Read the model definition and answer for the solid it produces. Units are mm, in the model's axes. A direction names the side the tool comes from. Give positions to 0.01 mm unless a question says otherwise; leave off trailing zeros. Loops run counter-clockwise (first coordinate to the right, second up) from the corner with the lowest first, then second, coordinate; pieces in that order, holes last. Notation, with made-up numbers: (9.25, -7) - (59.25, -7) arc R24 ccw to (59.25, 18) - close; hole circle Ø3 at (39.5, 45). An arc over 180 degrees is marked (long way). Write item = value, one per line. Start each with the question number.
from build123d import *
from build123d.topology import SkipClean

# Parameters (mm, degrees)
BOSS_EXTRUDE1_DEPTH             = 2
BOSS_EXTRUDE2_START             = -13.63
BOSS_EXTRUDE2_DEPTH             = 13.63
BOSS_EXTRUDE3_DEPTH             = 2
SKETCH5_W                       = 22.5
SKETCH5_H                       = 6.1
CUT_EXTRUDE1_DEPTH              = 28.613527482
BOSS_EXTRUDE4_REACH             = 29.614
SKETCH6_W                       = 22.5
SKETCH6_H                       = 3
BOSS_EXTRUDE4_DIRECTION_2_REACH = 29.614
FILLET1_R                       = 2


with BuildPart() as part:
    # Sketch1 → Boss-Extrude1 (new body)
    with BuildSketch(Plane(origin=(0, 0, 0), x_dir=(1, 0, 0), z_dir=(0, 1, 0))):
        with BuildLine():
            Line((2, 0), (20.5, 0))
            ThreePointArc((20.5, 0), (21.914213562, 0.585786438), (22.5, 2))
            Line((22.5, 2), (22.5, 5))
            ThreePointArc((22.5, 5), (21.914213562, 6.414213562), (20.5, 7))
            Line((20.5, 7), (2, 7))
            ThreePointArc((2, 7), (0.585786438, 6.414213562), (0, 5))
            Line((0, 5), (0, 2))
            ThreePointArc((0, 2), (0.585786438, 0.585786438), (2, 0))
        make_face()
    extrude(amount=BOSS_EXTRUDE1_DEPTH)

    # Sketch2 → Boss-Extrude2 (add)
    with SkipClean():  # the faces are left unmerged after this step: merging them gives an invalid solid
        with BuildSketch(Plane(origin=(0, 2, 0), x_dir=(1, 0, 0), z_dir=(0, 1, 0)).offset(BOSS_EXTRUDE2_START)):
            with BuildLine():
                Line((22.5, 5), (22.5, 2))
                ThreePointArc((22.5, 2), (22.202938637, 0.951191152), (21.4, 0.21394289))
                Line((21.4, 0.21394289), (21.4, 3.1))
                ThreePointArc((21.4, 3.1), (20.521320344, 5.221320344), (18.4, 6.1))
                Line((18.4, 6.1), (4.1, 6.1))
                ThreePointArc((4.1, 6.1), (1.978679656, 5.221320344), (1.1, 3.1))
                Line((1.1, 3.1), (1.1, 0.21394289))
                ThreePointArc((1.1, 0.21394289), (0.297061363, 0.951191152), (0, 2))
                Line((0, 2), (0, 5))
                ThreePointArc((0, 5), (0.585786438, 6.414213562), (2, 7))
                Line((2, 7), (20.5, 7))
                ThreePointArc((20.5, 7), (21.914213562, 6.414213562), (22.5, 5))
            make_face()
        extrude(amount=BOSS_EXTRUDE2_DEPTH)
    add(part.part.scale(1), mode=Mode.REPLACE)  # the faces are merged on a copy

    # Sketch4 → Boss-Extrude3 (add)
    with BuildSketch(Plane.XZ.offset(11.63)):
        with BuildLine():
            Line((20.5, -7), (2, -7))
            ThreePointArc((2, -7), (0.585786438, -6.414213562), (0, -5))
            Line((0, -5), (0, -9))
            ThreePointArc((0, -9), (0.585786438, -10.414213562), (2, -11))
            Line((2, -11), (20.5, -11))
            ThreePointArc((20.5, -11), (21.914213562, -10.414213562), (22.5, -9))
            Line((22.5, -9), (22.5, -5))
            ThreePointArc((22.5, -5), (21.914213562, -6.414213562), (20.5, -7))
        make_face()
    extrude(amount=-BOSS_EXTRUDE3_DEPTH)

    # Sketch5 → Cut-Extrude1 (cut, through all)
    with BuildSketch(Plane.XZ):
        with Locations((11.25, -3.05)):
            Rectangle(SKETCH5_W, SKETCH5_H)
    extrude(amount=CUT_EXTRUDE1_DEPTH, mode=Mode.SUBTRACT)

    # Boss-Extrude4: up to this face of the body (flat: up to its plane)
    boss_extrude4_end = Plane(part.part.faces().sort_by_distance((11.25, 2, -3.5))[0])
    # Sketch6 → Boss-Extrude4 (add, up to the picked face)
    with BuildSketch(Plane(origin=(0, -9.63, 0), x_dir=(1, 0, 0), z_dir=(0, 1, 0)), mode=Mode.PRIVATE) as boss_extrude4_sk1:
        with Locations((11.25, 6.5)):
            Rectangle(SKETCH6_W, SKETCH6_H)
    boss_extrude4_tool1 = split(extrude(boss_extrude4_sk1.sketch, amount=BOSS_EXTRUDE4_REACH, mode=Mode.PRIVATE), bisect_by=boss_extrude4_end, keep=Keep.BOTH, mode=Mode.PRIVATE)
    add(boss_extrude4_tool1.solids().sort_by(Axis((11.25, -9.63, -6.5), (0, 1, 0)))[0])

    # Boss-Extrude4 direction 2: up to this face of the body (flat: up to its plane)
    boss_extrude4_direction_2_end = Plane(part.part.faces().sort_by_distance((11.25, -11.63, -8.518311689))[0])
    # Sketch6 → Boss-Extrude4 direction 2 (add, up to the picked face)
    with BuildSketch(Plane(origin=(0, -9.63, 0), x_dir=(1, 0, 0), z_dir=(0, 1, 0)), mode=Mode.PRIVATE) as boss_extrude4_direction_2_sk1:
        with Locations((11.25, 6.5)):
            Rectangle(SKETCH6_W, SKETCH6_H)
    boss_extrude4_direction_2_tool1 = split(extrude(boss_extrude4_direction_2_sk1.sketch, amount=-BOSS_EXTRUDE4_DIRECTION_2_REACH, mode=Mode.PRIVATE), bisect_by=boss_extrude4_direction_2_end, keep=Keep.BOTH, mode=Mode.PRIVATE)
    add(boss_extrude4_direction_2_tool1.solids().sort_by(Axis((11.25, -9.63, -6.5), (0, -1, 0)))[0])

    # Fillet1
    fillet1_edges = [part.edges().sort_by_distance(p)[0] for p in [
        (11.25, -9.63, -8),
        (11.25, 2, -8),
    ]]
    fillet(fillet1_edges, radius=FILLET1_R)


solid = part.part
1. Consider line 1 along Y through (x, z) = (6, -10.25); line 2 along Z through (x, y) = (12.75, -6.5); line 3 along Y through (x, z) = (11.75, -0.25). Determine where each line is inside the solid, lowest interval first. Write a range as [from, to].
2. A cutting plane is placed at D-D on y = 1. Give the vertices of the cut face in (x, z).
3. Given P1, Ø8, axis at x = 8, y = -7.5, coming from the -Z side; P2, Ø4, axis at x = 19, y = -2, coming from the -Z side; P3, Ø6, axis at x = 17.5, z = -1.5, coming from the -Y side; P4, Ø0.5, axis at x = 14.5, z = -10.5, coming from the +Y side, each flat-ended and moving along its own axis, determine where each tip first touches the part or whether it passes through.
4. A cutting plane is placed at C-C on z = -4.25. Give the vertices of the cut face in (x, y), and give its area (3 significant figures).
5. A tool of negligible diameter and unlimited length cuts with its end or side. For faces 1 (the flat face through (11, -6, -5)), 2 (the flat face through (11.1, -9.63, -10.5)), 3 (the flat face through (11, 1, 0)), from which of +Z, -Z, +X, -X, +Y, -Y can it reach the whole face along a straight path? Write none if from no direction.
6. A cutting plane is placed at A-A on x = 3.75. Give the vertices of the cut face in (y, z).
7. A cutting plane is placed at B-B on y = -4.5. Give the vertices of the cut face in (x, z), and give its area (3 significant figures).
Reply:
q1.line_1 = [-11.63, -9.63]
q1.line_2 = [-8, -5]
q1.line_3 = [0, 2]
q2.outline = (0, -7.73) - (22.5, -7.73) - (22.5, -2) arc R2 ccw to (20.5, 0) - (2, 0) arc R2 ccw to (0, -2) - close
q3.P1 = -11
q3.P2 = -8
q3.P3 = 0
q3.P4 = -9.63
q4.outline = (0, 0) - (22.5, 0) - (22.5, 2) - (0, 2) - close
q4.area = 45.0 mm^2
q5.face_1 = +Z, +X, -X, -Y
q5.face_2 = -Z, +X, -X, +Y
q5.face_3 = +Z, +X, -X, +Y, -Y
q6.outline = (-11.63, -11) - (-9.63, -11) - (-9.63, -10) arc R2 cw to (-7.63, -8) - (0, -8) arc R2 ccw to (2, -6) - (2, 0) - (0, 0) - (0, -5) - (-11.63, -5) - close
q7.outline = (0, -8) - (22.5, -8) - (22.5, -5) - (0, -5) - close
q7.area = 67.5 mm^2
